Source: CAD feature listing. Evaluate the final solid. Frame: model axes, mm. A direction names the side the tool comes from. Round coordinates to 2 decimals unless told otherwise and drop trailing zeros. Write each loop counter-clockwise with the first axis right and the second up, starting at its lowest first coordinate (ties: lowest second). Pieces come first, ordered by that corner, then holes. Notation, with made-up numbers: M 29.5,-38 L 46.5,-38 A27 ccw 46.5,-16 Z; hole C -31.5,-22 d7. An arc over 180 degrees is marked long. Answer in a Markdown table with one row per item.
from build123d import *

# Parameters (mm, degrees)
EXTRUDE_1_DEPTH = 3


with BuildPart() as part:
    # 草图1 → 凸台-拉伸1 (new body)
    with BuildSketch(Plane.XY):
        with BuildLine():
            Line((2.5, 0), (64.6502, 0))
            ThreePointArc((64.6502, 0), (66.417966953, 0.732233047), (67.1502, 2.5))
            Line((67.1502, 2.5), (67.1502, 102.7498))
            ThreePointArc((67.1502, 102.7498), (66.417966953, 104.517566953), (64.6502, 105.2498))
            Line((64.6502, 105.2498), (2.5, 105.2498))
            ThreePointArc((2.5, 105.2498), (0.732233047, 104.517566953), (0, 102.7498))
            Line((0, 102.7498), (0, 2.5))
            ThreePointArc((0, 2.5), (0.732233047, 0.732233047), (2.5, 0))
        make_face()
        with BuildLine():
            Line((7.5, 100.2498), (59.6502, 100.2498))
            ThreePointArc((59.6502, 100.2498), (61.417966953, 99.517566953), (62.1502, 97.7498))
            Line((62.1502, 97.7498), (62.1502, 7.5))
            ThreePointArc((62.1502, 7.5), (61.417966953, 5.732233047), (59.6502, 5))
            Line((59.6502, 5), (7.5, 5))
            ThreePointArc((7.5, 5), (5.732233047, 5.732233047), (5, 7.5))
            Line((5, 7.5), (5, 97.7498))
            ThreePointArc((5, 97.7498), (5.732233047, 99.517566953), (7.5, 100.2498))
        make_face(mode=Mode.SUBTRACT)
    extrude(amount=EXTRUDE_1_DEPTH)


solid = part.part
Q1. Section C-C (x = 44.5). Return loops of the section in (y, z), and give its area (3 significant figures).
Solutions:
| item | result |
|---|---|
| outline | M 0,0 L 5,0 L 5,3 L 0,3 Z; M 100.25,0 L 105.25,0 L 105.25,3 L 100.25,3 Z |
| area | 30.0 mm2 |
Q2. Access query for faces 1 (the cylindrical face through (66.398, 0.713, 1.479)), 2 (the cylindrical face through (61.398, 99.537, 1.479)). Directions: +Z, -Z, +X, -X, +Y, -Y. A direction counts if a zero-diameter tool reaches every point of the face in a straight line with its end or side. Return the directions, or none.
Solutions:
| item | result |
|---|---|
| face 1 | +Z, -Z, +X, -Y |
| face 2 | +Z, -Z |
Q3. Section B-B (z = 1.65). Return loops of the section in (x, y).
Solutions:
| item | result |
|---|---|
| outline | M 0,2.5 A2.5 ccw 2.5,0 L 64.65,0 A2.5 ccw 67.15,2.5 L 67.15,102.75 A2.5 ccw 64.65,105.25 L 2.5,105.25 A2.5 ccw 0,102.75 Z; hole M 5,7.5 A2.5 ccw 7.5,5 L 59.65,5 A2.5 ccw 62.15,7.5 L 62.15,97.75 A2.5 ccw 59.65,100.25 L 7.5,100.25 A2.5 ccw 5,97.75 Z |
Q4. Section A-A (y = 45.5). Return loops of the section in (x, z).
Solutions:
| item | result |
|---|---|
| outline | M 0,0 L 5,0 L 5,3 L 0,3 Z; M 62.15,0 L 67.15,0 L 67.15,3 L 62.15,3 Z |
Q5. Pull-direction query (Y, two-part tool) for faces 3 (the cylindrical face through (66.437, 104.498, 1.479)), 4 (the flat face through (33, 100.25, 1)), 5 (the flat face through (4, 57, 3)), 6 (the cylindrical face through (61.437, 5.752, 1.479)); classes: pulls with the +Y half, pulls with the -Y half, needs draft (parallel to the pull), parting line crosses it, or undercut.
Solutions:
| item | result |
|---|---|
| face 3 | pulls with the +Y half |
| face 4 | undercut |
| face 5 | needs draft |
| face 6 | undercut |
Q6. Material intervals for probe 1 along Y at (x, z) = (22, 0.5); probe 2 along X at (y, z) = (15.5, 0.65); probe 3 along X at (y, z) = (6, 1.8), sorted ascending.
Solutions:
| item | result |
|---|---|
| probe 1 | y = 0 to 5, 100.25 to 105.25 |
| probe 2 | x = 0 to 5, 62.15 to 67.15 |
| probe 3 | x = 0 to 5.5, 61.65 to 67.15 |
